Part model, mm, in its own coordinate system. Give positions to 0.01 mm unless a question says otherwise; leave off trailing zeros. Order: outer loops, then holes, each group sorted by start corner. A loop starts at its lowest first (then second) coordinate and runs counter-clockwise, first axis right, second up. Notation, with made-up numbers: (-39.75, -2) - (-13.75, -2) arc R25 cw to (-13.75, 20) - close; hole circle Ø8 at (64, -21.5). An arc over 180 degrees is marked (long way). One line per item, written item: value.
```python
from build123d import *

# Parameters (mm, degrees)
SKETCH1_R           = 1.45
SKETCH1_R_2         = 2.95
BOSS_EXTRUDE1_DEPTH = 3
TROU_TARAUD_M1_61_D = 1.25


with BuildPart() as part:
    # Sketch1 → Boss-Extrude1 (new body)
    with BuildSketch(Plane.XY):
        with BuildLine():
            Line((15.5, 5.5), (-55, 5.5))
            ThreePointArc((-55, 5.5), (-60.5, 0), (-55, -5.5))
            Line((-55, -5.5), (15.5, -5.5))
            ThreePointArc((15.5, -5.5), (21, 0), (15.5, 5.5))
        make_face()
        with Locations((-55, 0)):
            Circle(SKETCH1_R, mode=Mode.SUBTRACT)
        Circle(SKETCH1_R_2, mode=Mode.SUBTRACT)
        with Locations((15.5, 0)):
            Circle(SKETCH1_R_2, mode=Mode.SUBTRACT)
    extrude(amount=BOSS_EXTRUDE1_DEPTH)

    # Trou taraudé M1.61 (through all)
    with Locations(Plane.XY.offset(3)):
        with Locations((7.75, 2.5), (-7.75, 2.5), (-50.5, 2.5), (-43, 2.5)):
            trou_taraud_m1_61 = Hole(TROU_TARAUD_M1_61_D / 2)

    # Mirror1: Trou taraudé M1.61 across plane
    add(trou_taraud_m1_61.mirror(Plane.ZX), mode=Mode.SUBTRACT)


solid = part.part
```
1) Slice it at D-D on x = 13.5. Write the cut outline in (y, z).
Answer:
outline: (-5.5, 0) - (-2.17, 0) - (-2.17, 3) - (-5.5, 3) - close; (2.17, 0) - (5.5, 0) - (5.5, 3) - (2.17, 3) - close
2) Drop a flat-ended pin along its axis: P1, Ø1, axis at y = -2.5, z = 1, coming from the -X side. Give the stop position or say it passes through.
Answer:
P1: stops at x = -60.12
3) Slice it at B-B on z = 1.4. Count the separate pieces of the cut face and the enclosed holes in it, then the cut area to 3 significant figures.
Answer:
separate pieces: 1
enclosed holes: 11
area: 799 mm2
4) Slice it at A-A on x = 0. Write the cut outline in (y, z), then the cut area to 3 significant figures.
Answer:
outline: (-5.5, 0) - (-2.95, 0) - (-2.95, 3) - (-5.5, 3) - close; (2.95, 0) - (5.5, 0) - (5.5, 3) - (2.95, 3) - close
area: 15.3 mm2
5) Two-plate mould, pull along Y, no slides. Class faces 1 (the face through (-19, 5.5, 1)), 2 (the face through (-43.577, 2.261, 1.479)), 3 (the face through (-20, 0, 0)): pulls with the +Y half, pulls with the -Y half, needs draft (parallel to the pull), parting line crosses it, or undercut.
Answer:
face 1: pulls with the +Y half
face 2: undercut
face 3: needs draft
6) Slice it at C-C on y = 0. Write the cut outline in (x, z).
Answer:
outline: (-60.5, 0) - (-56.45, 0) - (-56.45, 3) - (-60.5, 3) - close; (-53.55, 0) - (-2.95, 0) - (-2.95, 3) - (-53.55, 3) - close; (2.95, 0) - (12.55, 0) - (12.55, 3) - (2.95, 3) - close; (18.45, 0) - (21, 0) - (21, 3) - (18.45, 3) - close
7) Wall check: line 1 along Y through (x, z) = (-43, 1.8) (3 decimals); line 2 along X through (y, z) = (-1, 2.55); line 3 along X through (y, z) = (-1.5, 0.7). Give the ranges that are in metal, low to high. Write a range as [from, to].
Answer:
line 1: y = [-5.5, -3.125], [-1.875, 1.875], [3.125, 5.5]
line 2: x = [-60.41, -56.05], [-53.95, -2.78], [2.78, 12.72], [18.28, 20.91]
line 3: x = [-60.29, -2.54], [2.54, 12.96], [18.04, 20.79]
